Can you work these out from the model? Positions are in its coordinate system, mm. A direction names the side the tool comes from. Round coordinates to 2 decimals unless told otherwise and drop trailing zeros. Loops run counter-clockwise (first coordinate to the right, second up) from the corner with the lowest first, then second, coordinate; pieces in that order, holes last. Notation, with made-up numbers: (-22, 3.5) -> (-11, 3.5) arc R21 cw to (-11, 34.5) -> close; hole circle Ø8 at (82.25, 54). An arc over 180 degrees is marked (long way). Use a Markdown table: item, result.
from build123d import *

# Parameters (mm, degrees)
SKETCH1_R           = 9.5
BOSS_EXTRUDE1_DEPTH = 5


with BuildPart() as part:
    # Sketch1 → Boss-Extrude1 (new body)
    with BuildSketch(Plane.XY):
        Polygon((-35, 60), (-35, 55), (-25, 55), (-25, 60), (-5, 60), (-5, 55), (5, 55), (5, 60), (25, 60), (25, 55), (35, 55), (35, 60), (60, 60), (60, 40), (65, 40), (65, 30), (60, 30), (60, 10), (65, 10), (65, 0), (60, 0), (60, -20), (65, -20), (65, -30), (60, -30), (60, -60), (35, -60), (35, -65), (25, -65), (25, -60), (5, -60), (5, -65), (-5, -65), (-5, -60), (-25, -60), (-25, -65), (-35, -65), (-35, -60), (-60, -60), (-60, -30), (-65, -30), (-65, -20), (-60, -20), (-60, 0), (-65, 0), (-65, 10), (-60, 10), (-60, 30), (-65, 30), (-65, 40), (-60, 40), (-60, 60), align=None)
        with Locations((0, 35)):
            Circle(SKETCH1_R, mode=Mode.SUBTRACT)
    extrude(amount=BOSS_EXTRUDE1_DEPTH)


solid = part.part
1. Will these pins go through, and if not, where does the flat tip stop? pin 1 Ø1.5 at (y, z) = (-63, 3.5) entering from +X; pin 2 Ø2.5 at (x, z) = (63.5, 1.5) entering from +Y; pin 3 Ø10 at (x, y) = (49.5, -18) entering from -Z; pin 4 Ø1.5 at (x, z) = (47.5, 1.5) entering from -Y.
Answer sheet:
| item | result |
|---|---|
| pin 1 | stops at x = 35 |
| pin 2 | stops at y = 40 |
| pin 3 | stops at z = 0 |
| pin 4 | stops at y = -60 |
2. I want a section at A-A (y = 35). Please give me the cut outline in (x, z), plus the area to 3 significant figures.
Answer sheet:
| item | result |
|---|---|
| outline | (-65, 0) -> (-9.5, 0) -> (-9.5, 5) -> (-65, 5) -> close; (9.5, 0) -> (65, 0) -> (65, 5) -> (9.5, 5) -> close |
| area | 555 mm² |
3. I need wall thicknesses on line 1 (Y direction, x = 0, z = 3.6); line 2 (Y direction, x = -49.5, z = 1.35); line 3 (Y direction, x = 7, z = 3.05). Which ranges of each line are inside material? Lowest first, please.
Answer sheet:
| item | result |
|---|---|
| line 1 | y = -65 to 25.5, 44.5 to 55 |
| line 2 | y = -60 to 60 |
| line 3 | y = -60 to 28.58, 41.42 to 60 |
4. I want a section at B-B (x = 0). Please give me the cut outline in (y, z), plus the area to 3 significant figures.
Answer sheet:
| item | result |
|---|---|
| outline | (-65, 0) -> (25.5, 0) -> (25.5, 5) -> (-65, 5) -> close; (44.5, 0) -> (55, 0) -> (55, 5) -> (44.5, 5) -> close |
| area | 505 mm² |
5. Which directions (+Z, -Z, +X, -X, +Y, -Y) give clear straight access to the entire face, cutting with the end or side of a thin tool? Please do faces 1 (the flat face through (-63, 10, 2)), 2 (the flat face through (-25, -62, 2)), 3 (the flat face through (-47, -60, 2)), 4 (the flat face through (62, 10, 2)), 5 (the flat face through (0, 55, 2)).
Answer sheet:
| item | result |
|---|---|
| face 1 | +Z, -Z, -X |
| face 2 | +Z, -Z, -Y |
| face 3 | +Z, -Z, -X, -Y |
| face 4 | +Z, -Z, +X |
| face 5 | +Z, -Z, +Y |
6. If we mould it in two halves opening along X, with no side actions, what happens to faces 6 (the cylindrical face through (-1.24, 44.42, 2.46)), 7 (the flat face through (65, 35, 2)), 8 (the flat face through (63, -30, 2))? For each: +X half, -X half, draft (parallel to the pull), parting line (faces both ways), or undercut.
Answer sheet:
| item | result |
|---|---|
| face 6 | undercut |
| face 7 | +X half |
| face 8 | draft |
7. I want a section at C-C (y = 51). Please give me the cut outline in (x, z), plus the area to 3 significant figures.
Answer sheet:
| item | result |
|---|---|
| outline | (-60, 0) -> (60, 0) -> (60, 5) -> (-60, 5) -> close |
| area | 600 mm² |
